Can you work these out from the model? Positions are in its coordinate system, mm. A direction names the side the tool comes from. Give positions to 0.01 mm unless a question says otherwise; leave off trailing zeros. Loops run counter-clockwise (first coordinate to the right, second up) from the corner with the lowest first, then second, coordinate; pieces in that order, holes last. Notation, with made-up numbers: (-3, 46) - (46, 46) arc R26 ccw to (46, 65) - close; hole circle Ø9 at (63.25, 14). An arc over 180 degrees is marked (long way). Use a Markdown table: item, result. Add a question column.
```python
from build123d import *

# Parameters (mm, degrees)
F1_DEPTH = 76.2


with BuildPart() as f1:
    # F0 (on Top) → F1 (new body)
    with BuildSketch(Plane.XY):
        with BuildLine():
            Line((0, -0.762), (0, 0))
            Line((0, 0), (-47.625, 0))
            ThreePointArc((-47.625, 0), (-52.115128, 1.859872), (-53.975, 6.35))
            ThreePointArc((-53.975, 6.35), (-50.553519, 11.984384), (-43.976172, 11.546976))
            Line((-43.976172, 11.546976), (-42.47671, 10.494194))
            ThreePointArc((-42.47671, 10.494194), (-28.592771, 3.63091), (-13.286089, 1.27))
            Line((-13.286089, 1.27), (0, 1.27))
            Line((0, 1.27), (0, 2.032))
            Line((0, 2.032), (-13.286089, 2.032))
            ThreePointArc((-13.286089, 2.032), (-28.363171, 4.357496), (-42.038851, 11.117831))
            Line((-42.038851, 11.117831), (-43.538313, 12.170613))
            ThreePointArc((-43.538313, 12.170613), (-50.904941, 12.66051), (-54.737, 6.35))
            ThreePointArc((-54.737, 6.35), (-52.653943, 1.321057), (-47.625, -0.762))
            Line((-47.625, -0.762), (0, -0.762))
        make_face()
    extrude(amount=F1_DEPTH)


solid = f1.part
```
1. Suppose I cut it at C-C (z = 37). List the corners of the cut face in (x, y) for me (3 decimals).
2. Suppose I cut it at B-B (y = 4.25). List the corners of the cut face in (x, z) for me.
3. On a 3-axis mill with a long thin cutter (end or side, diameter ignored), from which of +Z, -Z, +X, -X, +Y, -Y can I reach the whole of each face in a straight line? I mean faces 1 (the face through (-24, -0.762, 38)), 2 (the face through (-28.8, 3.697, 37.567)), 3 (the face through (-7, 1.27, 38)). Say none if no direction works.
4. Suppose I cut it at A-A (x = -11). List the corners of the cut face in (y, z) for me, and give its area (3 significant figures).
5. If we mould it in two halves opening along Y, with no side actions, what happens to faces 4 (the face through (-7, 2.032, 38)), 5 (the face through (-29.5, 4.3, 76.2)), 6 (the face through (-43.2, 11, 37.6))? For each: released by +Y, released by -Y, zero draft, split by the parting line, or undercut.
6. Will these pins go through, and if not, where does the flat tip stop? P1, Ø10.5, axis at x = -10, z = 25.5, coming from the +Y side; P2, Ø6, axis at y = 1.5, z = 47.5, coming from the -X side; P3, Ø5, axis at y = 9, z = 50.5, coming from the -X side.
7. Please list where these lines run through material, in increasing order: line 1 along Y through (x, z) = (-7, 31.5); line 2 along Y through (x, z) = (-22.5, 32); line 3 along X through (y, z) = (10, 50). Write a range as [from, to].
Results below:
| question | item | result |
|---|---|---|
| 1 | outline | (-54.737, 6.35) arc R7.112 ccw to (-47.625, -0.762) - (0, -0.762) - (0, 0) - (-47.625, 0) arc R6.35 cw (long way) to (-43.976, 11.547) - (-42.477, 10.494) arc R50.8 ccw to (-13.286, 1.27) - (0, 1.27) - (0, 2.032) - (-13.286, 2.032) arc R50.038 cw to (-42.039, 11.118) - (-43.538, 12.171) arc R7.112 ccw to start |
| 2 | outline | (-54.42, 0) - (-53.62, 0) - (-53.62, 76.2) - (-54.42, 76.2) - close; (-30.43, 0) - (-28.02, 0) - (-28.02, 76.2) - (-30.43, 76.2) - close |
| 3 | face 1 | +Z, -Z, +X, -X, -Y |
| 3 | face 2 | +Z, -Z |
| 3 | face 3 | +Z, -Z, +X |
| 4 | outline | (-0.76, 0) - (0, 0) - (0, 76.2) - (-0.76, 76.2) - close; (1.27, 0) - (2.03, 0) - (2.03, 76.2) - (1.27, 76.2) - close |
| 4 | area | 116 mm² |
| 5 | face 4 | released by +Y |
| 5 | face 5 | zero draft |
| 5 | face 6 | undercut |
| 6 | P1 | y = 2.07 |
| 6 | P2 | x = -54.49 |
| 6 | P3 | x = -54.74 |
| 7 | line 1 | [-0.76, 0], [1.27, 2.03] |
| 7 | line 2 | [-0.76, 0], [2.11, 2.89] |
| 7 | line 3 | [-53.73, -52.82], [-41.76, -40.38] |
